Check sheet for the modelled part. Datum: model origin and axes. Units: mm. A direction names the side the tool comes from. Give positions to 0.01 mm unless a question says otherwise; leave off trailing zeros. Loops run counter-clockwise (first coordinate to the right, second up) from the corner with the lowest first, then second, coordinate; pieces in that order, holes last. Notation, with made-up numbers: (69, 83) -> (112, 83) arc R21 ccw to (112, 105) -> close; hole circle Ø2 at (24, -4.75). An arc over 180 degrees is marked (long way). Write each question's results on one line, items separated by ' | '. Start each with the question number.
1. Material ranges on L1, parallel to Z at x = 30, y = 0; L2, parallel to Z at x = 5.5, y = 75; L3, parallel to Z at x = 33.5, y = 86, recorded low to high. Write a range as from..to.
2. Cross-section at A-A on x = 5.5. Record the boundary of the cut face in (y, z).
3. Tool access check on faces 5 (the face through (31, 61, -8)), 6 (the face through (55.482, 92.871, 0.112)), 7 (the face through (15, 100, 11)), 8 (the face through (39, 62, 8)), 9 (the face through (31.059, -30.75, -21.464)). Record the directions out of +Z, -Z, +X, -X, +Y, -Y that give a thin tool (end or side, any length) a straight path to the whole face; none if there is none.
4. Cross-section at D-D on z = 48.5. Record the boundary of the cut face in (x, y).
5. Gauge pin test, flat ends, axial feed: pin 1 Ø1 at (x, z) = (45, 32.5) entering from +Y; pin 2 Ø2 at (x, y) = (13.5, 4) entering from -Z; pin 3 Ø1 at (x, y) = (22, 79) entering from +Z. Record the tip position at first contact, or that the pin passes through.
6. Cross-section at B-B on x = 33. Record the boundary of the cut face in (y, z), and give its area (3 significant figures).
7. Mould release check, pull along Y, two halves, no side actions. Record for faces 1 (the face through (7.888, 92.482, 57.871)), 2 (the face through (31.059, 23.846, 7.509)), 3 (the face through (8, 86, 40)), 4 (the face through (8, 51, 65)): +Y half, -Y half, draft (parallel to the pull), parting line (faces both ways), or undercut.
8. Cross-section at C-C on y = 73. Record the boundary of the cut face in (x, z).
from build123d import *

# Parameters (mm, degrees)
F0_R     = 25
F1_DEPTH = 63
F2_R     = 11
F3_DEPTH = 16
F4_R     = 10
F5_DEPTH = 100
F6_R     = 25


with BuildPart() as f1:
    # F0 (on Right) → F1 (new body)
    with BuildSketch(Plane.YZ):
        with BuildLine():
            Line((100, 8), (36.63673, 8))
            ThreePointArc((36.63673, 8), (-37.5, 0), (36.63673, -8))
            Line((36.63673, -8), (100, -8))
            Line((100, -8), (100, 8))
        make_face()
        Circle(F0_R, mode=Mode.SUBTRACT)
    extrude(amount=F1_DEPTH)

    # F2 (on face) → F3 (join)
    with BuildSketch(Plane(origin=(0, 0, 0), x_dir=(0, -1, 0), z_dir=(-1, 0, 0))):
        with BuildLine():
            Line((-27.5, 65), (-75, 65))
            ThreePointArc((-75, 65), (-92.67767, 57.67767), (-100, 40))
            Line((-100, 40), (-100, 8))
            Line((-100, 8), (-36.63673, 8))
            ThreePointArc((-36.63673, 8), (4.023221, 37.283558), (37.5, 0))
            ThreePointArc((37.5, 0), (18.461941, 45.961941), (-27.5, 65))
        make_face()
        with Locations((-75, 40)):
            Circle(F2_R, mode=Mode.SUBTRACT)
    extrude(amount=-F3_DEPTH)

    # F4 (on face) → F5 (cut)
    with BuildSketch(Plane.XY.offset(8)):
        with Locations((38, 75)):
            Circle(F4_R)
    extrude(amount=-F5_DEPTH, mode=Mode.SUBTRACT)

    # F6
    f6_edges = [f1.edges().sort_by_distance(p)[0] for p in [
        (63, 100, 0),
    ]]
    fillet(f6_edges, radius=F6_R)


solid = f1.part
Geometry says:
1) L1: -37.5..-25, 25..37.5 | L2: -8..29, 51..65 | L3: -8..8
2) outline: (-37.5, 0) arc R37.5 ccw to (36.64, -8) -> (100, -8) -> (100, 40) arc R25 ccw to (75, 65) -> (27.5, 65) arc R65 ccw to start; hole circle Ø50 at (0, 0); hole circle Ø22 at (75, 40)
3) face 5: -Z, +X, -X, +Y | face 6: +Z, -Z, +X, +Y | face 7: +Z, -Z, +X, -X, +Y | face 8: +Z, +X, +Y | face 9: +X
4) outline: (0, -15.78) -> (16, -15.78) -> (16, 68.02) -> (0, 68.02) -> close; (0, 81.98) -> (16, 81.98) -> (16, 98.51) -> (0, 98.51) -> close
5) pin 1: y = 19.55 | pin 2: z = -37.38 | pin 3: z = 8
6) outline: (36.64, -8) -> (66.34, -8) -> (66.34, 8) -> (36.64, 8) arc R37.5 ccw (long way) to start; (83.66, -8) -> (100, -8) -> (100, 8) -> (83.66, 8) -> close; hole circle Ø50 at (0, 0) | area: 3,180 mm^2
7) face 1: +Y half | face 2: undercut | face 3: undercut | face 4: draft
8) outline: (0, -8) -> (28.2, -8) -> (28.2, 8) -> (16, 8) -> (16, 29.18) -> (0, 29.18) -> close; (0, 50.82) -> (16, 50.82) -> (16, 65) -> (0, 65) -> close; (47.8, -8) -> (63, -8) -> (63, 8) -> (47.8, 8) -> close
